Can you work these out from the model? Positions are in its coordinate system, mm. A direction names the side the tool comes from. Round coordinates to 2 decimals unless told otherwise and drop trailing zeros. Order: outer loops, then holes, each group sorted by start corner. A loop starts at its lowest first (then second) coordinate and runs counter-clockwise, first axis right, second up. Notation, with made-up numbers: (-25, 7.5) - (10, 7.5) arc R20 ccw to (10, 43.5) - close; hole circle Ø2 at (84, 69.5). An arc over 180 degrees is marked (long way). Write item = value, one per line.
from build123d import *

# Parameters (mm, degrees)
SKETCH1_W           = 10
SKETCH1_H           = 40
BOSS_EXTRUDE1_DEPTH = 3
SKETCH2_R           = 1.7
CUT_EXTRUDE1_DEPTH  = 7
SKETCH3_W           = 10
SKETCH3_H           = 10
BOSS_EXTRUDE2_DEPTH = 25
SKETCH7_R           = 1
BOSS_EXTRUDE3_DEPTH = 5
SKETCH9_R           = 1.5
BOSS_EXTRUDE4_DEPTH = 9
SKETCH10_R          = 0.875
BOSS_EXTRUDE5_DEPTH = 2
FILLET1_R           = 0.5
CHAMFER1_SIZE       = 7.5
CHAMFER2_SIZE       = 7
SKETCH11_W          = 10
SKETCH11_H          = 2.819588602
CUT_EXTRUDE2_DEPTH  = 10


with BuildPart() as part:
    # Sketch1 → Boss-Extrude1 (new body)
    with BuildSketch(Plane.XY):
        with Locations((5, 20)):
            Rectangle(SKETCH1_W, SKETCH1_H)
    extrude(amount=BOSS_EXTRUDE1_DEPTH)

    # Sketch2 → Cut-Extrude1 (cut)
    with BuildSketch(Plane.XY.offset(3)):
        with Locations((5, 37.5)):
            Circle(SKETCH2_R)
        with Locations((5, 5)):
            Circle(SKETCH2_R)
    extrude(amount=-CUT_EXTRUDE1_DEPTH, mode=Mode.SUBTRACT)

    # Sketch3 → Boss-Extrude2 (add)
    with BuildSketch(Plane.XY.offset(3)):
        with Locations((5, 20)):
            Rectangle(SKETCH3_W, SKETCH3_H)
    extrude(amount=BOSS_EXTRUDE2_DEPTH)

    # Sketch7 → Boss-Extrude3 (add)
    with BuildSketch(Plane.XY.offset(28)):
        Polygon((-7.5, 8), (17.5, 8), (17.5, 32), (17.5, 35), (-7.5, 35), (-7.5, 32), align=None)
        with Locations((-5.5, 20)):
            Circle(SKETCH7_R, mode=Mode.SUBTRACT)
        with Locations((15.5, 20)):
            Circle(SKETCH7_R, mode=Mode.SUBTRACT)
        with Locations((-5.5, 32.5)):
            Circle(SKETCH7_R, mode=Mode.SUBTRACT)
        with Locations((15.5, 32.5)):
            Circle(SKETCH7_R, mode=Mode.SUBTRACT)
    extrude(amount=BOSS_EXTRUDE3_DEPTH)

    # Sketch9 → Boss-Extrude4 (add)
    with BuildSketch(Plane(origin=(0, 0, 28), x_dir=(-1, 0, 0), z_dir=(0, 0, -1))):
        with Locations((5.5, 32.5)):
            Circle(SKETCH9_R)
        with Locations((-15.5, 32.5)):
            Circle(SKETCH9_R)
        with Locations((-15.5, 20)):
            Circle(SKETCH9_R)
        with Locations((5.5, 20)):
            Circle(SKETCH9_R)
    extrude(amount=-BOSS_EXTRUDE4_DEPTH)

    # Sketch10 → Boss-Extrude5 (add)
    with BuildSketch(Plane.XY.offset(37)):
        with Locations((-5.5, 32.5)):
            Circle(SKETCH10_R)
        with Locations((15.5, 32.5)):
            Circle(SKETCH10_R)
        with Locations((15.5, 20)):
            Circle(SKETCH10_R)
        with Locations((-5.5, 20)):
            Circle(SKETCH10_R)
    extrude(amount=BOSS_EXTRUDE5_DEPTH)

    # Fillet1
    fillet1_edges = [part.edges().sort_by_distance(p)[0] for p in [
        (-6.375, 20, 39),
        (14.625, 20, 39),
        (14.625, 32.5, 39),
        (-6.375, 32.5, 39),
    ]]
    fillet(fillet1_edges, radius=FILLET1_R)

    # Chamfer1
    chamfer1_edges = [part.edges().sort_by_distance(p)[0] for p in [
        (0, 20, 28),
        (10, 20, 28),
    ]]
    chamfer(chamfer1_edges, length=CHAMFER1_SIZE - 0.0001)  # a hair under: the kernel refuses the full size

    # Chamfer2
    chamfer2_edges = [part.edges().sort_by_distance(p)[0] for p in [
        (5, 15, 28),
        (5, 25, 28),
    ]]
    chamfer(chamfer2_edges, length=CHAMFER2_SIZE - 0.0001)  # a hair under: the kernel refuses the full size

    # Sketch11 → Cut-Extrude2 (cut)
    with BuildSketch(Plane.XY.offset(33)):
        with Locations((5, 9.409794301)):
            Rectangle(SKETCH11_W, SKETCH11_H)
    extrude(amount=-CUT_EXTRUDE2_DEPTH, mode=Mode.SUBTRACT)


solid = part.part
(1) If we section it at B-B (x = 5): Write out the boundary of the cut face in (y, z).
Computed:
outline = (0, 0) - (3.3, 0) - (3.3, 3) - (0, 3) - close; (6.7, 0) - (35.8, 0) - (35.8, 3) - (25, 3) - (25, 21) - (32, 28) - (35, 28) - (35, 33) - (10.82, 33) - (10.82, 25.18) - (15, 21) - (15, 3) - (6.7, 3) - close; (39.2, 0) - (40, 0) - (40, 3) - (39.2, 3) - close
(2) On a 3-axis mill with a long thin cutter (end or side, diameter ignored), from which of +Z, -Z, +X, -X, +Y, -Y can I reach the whole of each face in a straight line? I mean faces 4 (the face through (5, 29, 25)), 5 (the face through (-6.5, 32.2, 37)), 6 (the face through (5, 10.82, 29)). Say none if no direction works.
Computed:
face_4 = +X, -X, +Y
face_5 = +Z
face_6 = +Z, -Y
(3) If we section it at D-D (x = 9.25): Write out the boundary of the cut face in (y, z), plus the area to 3 significant figures.
Computed:
outline = (0, 0) - (40, 0) - (40, 3) - (25, 3) - (25, 21) - (32, 28) - (35, 28) - (35, 33) - (10.82, 33) - (10.82, 25.18) - (15, 21) - (15, 3) - (0, 3) - close
area = 536 mm^2
(4) If we section it at C-C (z = 35.5): Write out the boundary of the cut face in (x, y).
Computed:
outline = circle Ø3 at (-5.5, 20); circle Ø3 at (-5.5, 32.5); circle Ø3 at (15.5, 20); circle Ø3 at (15.5, 32.5)
(5) Will these pins go through, and if not, where does the flat tip stop? P1, Ø3, axis at x = 14.5, y = 29, coming from the -Z side; P2, Ø3, axis at x = 7.5, y = 20, coming from the +Z side; P3, Ø16.5, axis at y = 20.5, z = 11, coming from the -X side.
Computed:
P1 = 23.94
P2 = 33
P3 = 0
(6) If I drill on line 1 (Y direction, x = 5, z = 1.3); line 2 (Z direction, x = 3.25, y = 8.5); line 3 (X direction, y = 18, z = 13), over which ranges is the centre line in solid material (lowest first)? Write a range as from..to.
Computed:
line_1 = 0..3.3, 6.7..35.8, 39.2..40
line_2 = 0..3
line_3 = 0..10
(7) If we section it at A-A (y = 37.5): Write out the boundary of the cut face in (x, z).
Computed:
outline = (0, 0) - (3.3, 0) - (3.3, 3) - (0, 3) - close; (6.7, 0) - (10, 0) - (10, 3) - (6.7, 3) - close
(8) Thinking about a two-plate mould opening in Y: for faces 1 (the face through (15.825, 31.036, 34.972)), 2 (the face through (14.5, 19.8, 25)), 3 (the face through (5, 40, 1)), which applies, +Y half, -Y half, draft (parallel to the pull), parting line (faces both ways), or undercut?
Computed:
face_1 = undercut
face_2 = draft
face_3 = +Y half
